CAD build for the part. Positions are in the model's coordinates, mm. A direction names the side the tool comes from. Give positions to 0.01 mm unless a question says otherwise; leave off trailing zeros. Write each loop counter-clockwise with the first axis right and the second up, starting at its lowest first coordinate (ties: lowest second). Pieces come first, ordered by that corner, then holes. Notation, with made-up numbers: (-29, -12) - (23, -12) arc R29 ccw to (23, 23) - close; hole circle Ø6 at (-12, 20). An arc over 180 degrees is marked (long way). Answer as a JSON object with one key per item and string values.
from build123d import *

# Parameters (mm, degrees)
SKETCH3_R           = 1.4224
SKETCH3_W           = 6.35
SKETCH3_H           = 6.35
BOSS_EXTRUDE1_DEPTH = 6.35
FILLET1_R           = 10.16
FILLET2_R           = 27.94


with BuildPart() as part:
    # Sketch3 → Boss-Extrude1 (new body)
    with BuildSketch(Plane(origin=(0, 0, 0), x_dir=(1, 0, 0), z_dir=(0, 1, 0))):
        with BuildLine():
            Line((182.88, 0), (0, 0))
            Line((0, 0), (0, 262.339276313))
            Line((0, 262.339276313), (182.88, 262.339276313))
            Line((182.88, 262.339276313), (182.88, 169.269638157))
            ThreePointArc((182.88, 169.269638157), (144.78, 131.169638157), (182.88, 93.069638157))
            Line((182.88, 93.069638157), (182.88, 0))
        make_face()
        with Locations(Location((57.15, 38.1, 0), (0, 0, 270))):
            Circle(SKETCH3_R, mode=Mode.SUBTRACT)
        with Locations(Location((57.15, 114.3, 0), (0, 0, 270))):
            Circle(SKETCH3_R, mode=Mode.SUBTRACT)
        with Locations(Location((125.73, 114.3, 0), (0, 0, 90))):
            Circle(SKETCH3_R, mode=Mode.SUBTRACT)
        with Locations(Location((125.73, 38.1, 0), (0, 0, 90))):
            Circle(SKETCH3_R, mode=Mode.SUBTRACT)
        with Locations(Location((69.85, 151.157668748, 0), (0, 0, 270))):
            Circle(SKETCH3_R, mode=Mode.SUBTRACT)
        with Locations(Location((69.85, 219.737668748, 0), (0, 0, 270))):
            Circle(SKETCH3_R, mode=Mode.SUBTRACT)
        with Locations(Location((113.03, 151.157668748, 0), (0, 0, 90))):
            Circle(SKETCH3_R, mode=Mode.SUBTRACT)
        with Locations(Location((113.03, 219.737668748, 0), (0, 0, 90))):
            Circle(SKETCH3_R, mode=Mode.SUBTRACT)
        with Locations(Location((113.03, 42.601607565, 0), (0, 0, 270))):
            Circle(SKETCH3_R, mode=Mode.SUBTRACT)
        with Locations(Location((113.03, 111.181607565, 0), (0, 0, 270))):
            Circle(SKETCH3_R, mode=Mode.SUBTRACT)
        with Locations(Location((69.85, 111.181607565, 0), (0, 0, 90))):
            Circle(SKETCH3_R, mode=Mode.SUBTRACT)
        with Locations(Location((69.85, 42.601607565, 0), (0, 0, 90))):
            Circle(SKETCH3_R, mode=Mode.SUBTRACT)
        with Locations(Location((125.73, 148.039276313, 0), (0, 0, 270))):
            Circle(SKETCH3_R, mode=Mode.SUBTRACT)
        with Locations(Location((125.73, 224.239276313, 0), (0, 0, 270))):
            Circle(SKETCH3_R, mode=Mode.SUBTRACT)
        with Locations(Location((57.15, 224.239276313, 0), (0, 0, 90))):
            Circle(SKETCH3_R, mode=Mode.SUBTRACT)
        with Locations(Location((57.15, 148.039276313, 0), (0, 0, 90))):
            Circle(SKETCH3_R, mode=Mode.SUBTRACT)
        with Locations((22.225, 13.212735966)):
            Rectangle(SKETCH3_W, SKETCH3_H, mode=Mode.SUBTRACT)
        with Locations((160.655, 13.212735966)):
            Rectangle(SKETCH3_W, SKETCH3_H, mode=Mode.SUBTRACT)
        with Locations((160.655, 249.126540348)):
            Rectangle(SKETCH3_W, SKETCH3_H, mode=Mode.SUBTRACT)
        with Locations((22.225, 249.126540348)):
            Rectangle(SKETCH3_W, SKETCH3_H, mode=Mode.SUBTRACT)
    extrude(amount=BOSS_EXTRUDE1_DEPTH)

    # Fillet1
    fillet1_edges = [part.edges().sort_by_distance(p)[0] for p in [
        (0, 3.175, -262.339276313),
        (182.88, 3.175, -262.339276313),
        (182.88, 3.175, 0),
        (0, 3.175, 0),
    ]]
    fillet(fillet1_edges, radius=FILLET1_R)

    # Fillet2
    fillet2_edges = [part.edges().sort_by_distance(p)[0] for p in [
        (182.88, 3.175, -169.269638157),
        (182.88, 3.175, -93.069638157),
    ]]
    fillet(fillet2_edges, radius=FILLET2_R)


solid = part.part
(1) 3-axis set-ups, long thin cutter, end or side, ignore diameter. For faces 5 (the face through (22, 3, -10.038)), 6 (the face through (178.627, 3.219, -86.15)), 7 (the face through (93, 6.35, -133)): which of +Z, -Z, +X, -X, +Y, -Y reach the whole face in a straight line?
Answer key:
{"face 5": "+Y, -Y", "face 6": "+X, +Y, -Y", "face 7": "+Z, -Z, +X, -X, +Y"}
(2) Probe L1, parallel to Z at x = 125.73, y = 3; L2, parallel to Z at x = 69.85, y = 2.75; L3, parallel to X at y = 1, z = -219. List the from-to ranges inside material, lowest first. Write a range as [from, to].
Answer key:
{"L1": "z = [-262.34, -225.66], [-222.82, -149.46], [-146.62, -115.72], [-112.88, -39.52], [-36.68, 0]", "L2": "z = [-262.34, -221.16], [-218.32, -152.58], [-149.74, -112.6], [-109.76, -44.02], [-41.18, 0]", "L3": "x = [0, 68.63], [71.07, 111.81], [114.25, 182.88]"}
(3) Saw through at A-A, the plane z = -171. Give the cut face in (x, y), and give its area (3 significant figures).
Answer key:
{"outline": "(0, 0) - (174.44, 0) - (174.44, 6.35) - (0, 6.35) - close", "area": "1,110 mm²"}
(4) Pull direction Z, two halves, no side cores. Call faces 1 (the face through (93, 3, 0)), 2 (the face through (179.825, 3.219, -259.442)), 3 (the face through (161, 3, -252.302)), 4 (the face through (0, 3, -129)): pulls with the +Z half, pulls with the -Z half, needs draft (parallel to the pull), parting line crosses it, or undercut.
Answer key:
{"face 1": "pulls with the +Z half", "face 2": "pulls with the -Z half", "face 3": "undercut", "face 4": "needs draft"}
